from build123d import *

# Parameters (mm, degrees)
SCHIZZO1_R                   = 60.25
ESTRUSIONE_ESTRUSIONE1_DEPTH = 1.3
SCHIZZO1_6_R                 = 64.5
SCHIZZO1_6_R_2               = 60.25
ESTRUSIONE_ESTRUSIONE2_DEPTH = 5
ESTRUSIONE_ESTRUSIONE3_START = 5
SCHIZZO2_R                   = 60.25
ESTRUSIONE_ESTRUSIONE3_DEPTH = 5
SCHIZZO4_R                   = 2.2
TAGLIO_ESTRUSIONE1_DEPTH     = 22.55
SCHIZZO5_R                   = 2.2
SCHIZZO5_R_2                 = 2.063369246
TAGLIO_ESTRUSIONE2_DEPTH     = 92.35370819
SCHIZZO6_R                   = 3.55
TAGLIO_ESTRUSIONE3_DEPTH     = 3
TAGLIO_ESTRUSIONE4_DEPTH     = 92.434074611
TAGLIO_ESTRUSIONE5_DEPTH     = 92.434074611
SCHIZZO19_R                  = 2.2
TAGLIO_ESTRUSIONE6_DEPTH     = 92.434074611
SCHIZZO21_W                  = 23.016895474
SCHIZZO21_H                  = 3.000921099
TAGLIO_ESTRUSIONE7_DEPTH     = 92.434074611
SCHIZZO23_W                  = 21.797647442
SCHIZZO23_H                  = 17.331114079
TAGLIO_ESTRUSIONE8_DEPTH     = 92.434074611
SCHIZZO24_W                  = 6.255388186
SCHIZZO24_H                  = 0.117454314
TAGLIO_ESTRUSIONE9_DEPTH     = 92.35370819
SCHIZZO25_W                  = 6.255388186
SCHIZZO25_H                  = 0.117454314
TAGLIO_ESTRUSIONE10_DEPTH    = 92.434074611


with BuildPart() as part:
    # Schizzo1 → Estrusione-Estrusione1 (new body)
    with BuildSketch(Plane.XY):
        Circle(SCHIZZO1_R)
    extrude(amount=ESTRUSIONE_ESTRUSIONE1_DEPTH)



with BuildPart() as body_2:
    # Schizzo1_6 → Estrusione-Estrusione2 (new body)
    with BuildSketch(Plane.XY):
        Circle(SCHIZZO1_6_R)
        Circle(SCHIZZO1_6_R_2, mode=Mode.SUBTRACT)
    extrude(amount=-ESTRUSIONE_ESTRUSIONE2_DEPTH)


with BuildPart() as part_1:
    add(part.part)

    add(body_2.part)  # Estrusione-Estrusione3 merges body 2
    # Schizzo2 → Estrusione-Estrusione3 (add)
    with BuildSketch(Plane(origin=(0, 0, 0), x_dir=(-1, 0, 0), z_dir=(0, 0, -1)).offset(ESTRUSIONE_ESTRUSIONE3_START)):
        with Locations(Location((0, 0, 0), (0, 0, 180))):
            Circle(SCHIZZO2_R)
    extrude(amount=-ESTRUSIONE_ESTRUSIONE3_DEPTH)

    # Schizzo4 → Taglio-Estrusione1 (cut)
    with BuildSketch(Plane.XY):
        with Locations((-38.215953468, 42.185917173)):
            Circle(SCHIZZO4_R)
        with Locations((42.295854852, 38.002469644)):
            Circle(SCHIZZO4_R)
        with Locations((-42.258051235, -38.212951628)):
            Circle(SCHIZZO4_R)
    extrude(amount=TAGLIO_ESTRUSIONE1_DEPTH, mode=Mode.SUBTRACT)

    # Schizzo5 → Taglio-Estrusione2 (cut, through all)
    with BuildSketch(Plane.XY):
        with Locations((42.295854852, 38.002469644)):
            Circle(SCHIZZO5_R)
        with Locations((-38.215953468, 42.185917173)):
            Circle(SCHIZZO5_R_2)
        with Locations((-42.258051235, -38.212951628)):
            Circle(SCHIZZO5_R)
    extrude(amount=-TAGLIO_ESTRUSIONE2_DEPTH, mode=Mode.SUBTRACT)

    # Schizzo6 → Taglio-Estrusione3 (cut)
    with BuildSketch(Plane(origin=(0, 0, -5), x_dir=(-1, 0, 0), z_dir=(0, 0, -1))):
        with Locations((-42.295854852, 38.002469644)):
            Circle(SCHIZZO6_R)
        with Locations((38.215953468, 42.185917173)):
            Circle(SCHIZZO6_R)
        with Locations((42.258051235, -38.212951628)):
            Circle(SCHIZZO6_R)
    extrude(amount=-TAGLIO_ESTRUSIONE3_DEPTH, mode=Mode.SUBTRACT)

    # Schizzo16 → Taglio-Estrusione4 (cut, through all)
    with BuildSketch(Plane.XY.offset(1.3)):
        with BuildLine():
            Line((-32.928448826, 14.986032767), (-25.1744035, 14.986032767))
            Line((-25.1744035, 14.986032767), (-25.1744035, -0.412845979))
            Line((-25.1744035, -0.412845979), (-8.028134258, -0.412845979))
            Line((-8.028134258, -0.412845979), (-6.936015198, 0.679273081))
            Line((-6.936015198, 0.679273081), (-6.936015198, 13.042885081))
            ThreePointArc((-6.936015198, 13.042885081), (-6.332478846, 14.499950729), (-4.875413198, 15.103487081))
            Line((-4.875413198, 15.103487081), (3.18719168, 15.103487081))
            ThreePointArc((3.18719168, 15.103487081), (3.567159045, 15.553378343), (4.131478144, 15.721667681))
            Line((4.131478144, 15.721667681), (23.016895474, 15.721667681))
            ThreePointArc((23.016895474, 15.721667681), (23.745428298, 15.419899505), (24.047196474, 14.691366681))
            Line((24.047196474, 14.691366681), (24.047196474, -5.607623621))
            ThreePointArc((24.047196474, -5.607623621), (23.745428298, -6.336156444), (23.016895474, -6.637924621))
            Line((23.016895474, -6.637924621), (-32.928448826, -6.637924621))
            Line((-32.928448826, -6.637924621), (-32.928448826, 14.986032767))
        make_face()
    extrude(amount=-TAGLIO_ESTRUSIONE4_DEPTH, mode=Mode.SUBTRACT)

    # Schizzo18 → Taglio-Estrusione5 (cut, through all)
    with BuildSketch(Plane(origin=(0, 0, -5), x_dir=(-1, 0, 0), z_dir=(0, 0, -1))):
        Polygon((30.728647486, 5.653371487), (32.000647486, 6.387761029), (44.000647486, 6.387761029), (45.20554645, 5.664349962), (45.156092105, 2.475905944), (44.000647486, 1.737761029), (32.000647486, 1.738981944), (30.728647486, 2.473371487), align=None)
    extrude(amount=-TAGLIO_ESTRUSIONE5_DEPTH, mode=Mode.SUBTRACT)

    # Schizzo19 → Taglio-Estrusione6 (cut, through all)
    with BuildSketch(Plane.XY.offset(1.3)):
        with Locations((-47.096963083, -2.216170811)):
            Circle(SCHIZZO19_R)
        with Locations((-47.096963083, 9.498765652)):
            Circle(SCHIZZO19_R)
        with Locations((-24.967055149, -19.916033665)):
            Circle(SCHIZZO19_R)
        with Locations((-11.036476343, -19.916033665)):
            Circle(SCHIZZO19_R)
    extrude(amount=-TAGLIO_ESTRUSIONE6_DEPTH, mode=Mode.SUBTRACT)

    # Schizzo21 → Taglio-Estrusione7 (cut, through all)
    with BuildSketch(Plane(origin=(0, 0, -5), x_dir=(-1, 0, 0), z_dir=(0, 0, -1))):
        with Locations((-11.508447737, -8.138385171)):
            Rectangle(SCHIZZO21_W, SCHIZZO21_H)
    extrude(amount=-TAGLIO_ESTRUSIONE7_DEPTH, mode=Mode.SUBTRACT)

    # Schizzo23 → Taglio-Estrusione8 (cut, through all)
    with BuildSketch(Plane(origin=(0, 0, -5), x_dir=(-1, 0, 0), z_dir=(0, 0, -1))):
        with Locations((15.774236919, 6.437930042)):
            Rectangle(SCHIZZO23_W, SCHIZZO23_H)
    extrude(amount=-TAGLIO_ESTRUSIONE8_DEPTH, mode=Mode.SUBTRACT)

    # Schizzo24 → Taglio-Estrusione9 (cut, through all)
    with BuildSketch(Plane.XY):
        with Locations((-29.800754733, 15.044759924)):
            Rectangle(SCHIZZO24_W, SCHIZZO24_H)
    extrude(amount=-TAGLIO_ESTRUSIONE9_DEPTH, mode=Mode.SUBTRACT)

    # Schizzo25 → Taglio-Estrusione10 (cut, through all)
    with BuildSketch(Plane.XY.offset(1.3)):
        with Locations((-29.800754733, 15.044759924)):
            Rectangle(SCHIZZO25_W, SCHIZZO25_H)
    extrude(amount=-TAGLIO_ESTRUSIONE10_DEPTH, mode=Mode.SUBTRACT)


solid = part_1.part
Check sheet for the modelled part. Datum: model origin and axes. Units: mm. A direction names the side the tool comes from. Coordinates: 2 decimals unless noted, no trailing zeros. Loops run counter-clockwise (first coordinate to the right, second up) from the corner with the lowest first, then second, coordinate; pieces in that order, holes last. Notation, with made-up numbers: (82.25, 18.5) -> (117.25, 18.5) arc R7 ccw to (117.25, 31.5) -> close; hole circle Ø6 at (11.25, 53.5). An arc over 180 degrees is marked (long way). Write item = value, one per line. Start each with the question number.
1. Depth check by flat-ended pin: P1, Ø2, axis at x = -42, y = -39.5, coming from the -Z side; P2, Ø2.5, axis at x = 42.3, y = 38, coming from the +Z side; P3, Ø1.5, axis at y = -8.5, z = -0.5, coming from the +X side; P4, Ø5, axis at x = -47.1, y = 9.5, coming from the -Z side. Enter the tip coordinate at first touch or a pass-through.
2. Draft check along X on faces 1 (the cylindrical face through (-47.812, -36.661, 0.641)), 2 (the flat face through (-1, -13, 1.3)), 3 (the cylindrical face through (41.819, 35.855, -0.327)), 4 (the flat face through (-42, -41, -2)). Enter one of: released by +X, released by -X, zero draft, split by the parting line, or undercut.
3. Material ranges on line 1 (Y direction, x = -23, z = -4); line 2 (Y direction, x = -33, z = 0.5); line 3 (Y direction, x = 22, z = -4.5), recorded low to high.
4. Section check A-A on x = 15. Record the cut outline in (y, z), then the cut area to 3 significant figures.
5. Section check B-B on x = -11. Record the cut outline in (y, z), then the cut area to 3 significant figures.
6. Tool access check on faces 5 (the flat face through (-41, 42, -2)), 6 (the flat face through (-38, 6.388, -2)), 7 (the cylindrical face through (-39.84, 43.67, 0.64)). Record the directions out of +Z, -Z, +X, -X, +Y, -Y that give a thin tool (end or side, any length) a straight path to the whole face; none if there is none.
7. Section check C-C on x = 51. Record the cut outline in (y, z).
Responses:
q1.P1 = -2
q1.P2 = through
q1.P3 = 64.03
q1.P4 = -5
q2.face_1 = split by the parting line
q2.face_2 = zero draft
q2.face_3 = undercut
q2.face_4 = undercut
q3.line_1 = -60.26 to -20.9, -18.93 to -6.64, 15.1 to 60.26
q3.line_2 = -50.41 to 1.74, 6.39 to 50.41
q3.line_3 = -60.63 to -9.64, 15.72 to 60.63
q4.outline = (-62.73, -5) -> (-9.64, -5) -> (-9.64, 1.3) -> (-58.35, 1.3) -> (-58.35, 0) -> (-62.73, 0) -> close; (15.72, -5) -> (62.73, -5) -> (62.73, 0) -> (58.35, 0) -> (58.35, 1.3) -> (15.72, 1.3) -> close
q4.area = 619 mm2
q5.outline = (-63.56, -5) -> (-22.12, -5) -> (-22.12, 1.3) -> (-59.24, 1.3) -> (-59.24, 0) -> (-63.56, 0) -> close; (-17.72, -5) -> (-6.64, -5) -> (-6.64, 1.3) -> (-17.72, 1.3) -> close; (15.1, -5) -> (63.56, -5) -> (63.56, 0) -> (59.24, 0) -> (59.24, 1.3) -> (15.1, 1.3) -> close
q5.area = 625 mm2
q6.face_5 = -Z
q6.face_6 = +Z, -Z
q6.face_7 = +Z
q7.outline = (-39.49, -5) -> (39.49, -5) -> (39.49, 0) -> (32.08, 0) -> (32.08, 1.3) -> (-32.08, 1.3) -> (-32.08, 0) -> (-39.49, 0) -> close
